Design review of the part built by this model. Coordinates are the model's own, in mm. Face numbers are marked on the shaded views. A direction names the side the tool comes from. Coordinates: 2 decimals unless noted, no trailing zeros. Loops run counter-clockwise (first coordinate to the right, second up) from the corner with the lowest first, then second, coordinate; pieces in that order, holes last. Notation, with made-up numbers: M 39,51.25 L 92,51.25 A37 cw 92,90.25 Z; hole C -4,18.25 d6. An arc over 180 degrees is marked long. Write item = value, one per line. Start each with the question number.
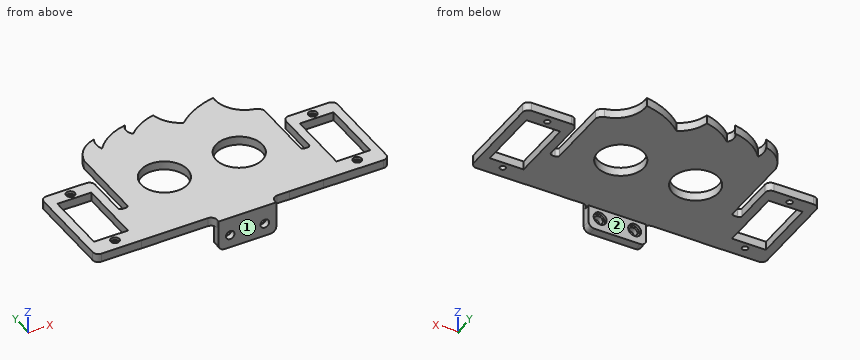
```python
from build123d import *

# Parameters (mm, degrees)
MODEL_R                 = 8.05
MODEL_R_2               = 1
MODEL_W                 = 11.8
MODEL_H                 = 22.5
SALIENTE_EXTRUIR1_DEPTH = 3
CROQUIS1_W              = 19.999999999
CROQUIS1_H              = 3
SALIENTE_EXTRUIR2_DEPTH = 8
CROQUIS2_R              = 1.5
CORTAR_EXTRUIR1_DEPTH   = 3
REDONDEO2_R             = 2
CROQUIS3_R              = 1.5
CORTAR_EXTRUIR2_DEPTH   = 1
CROQUIS4_R              = 2.25
CORTAR_EXTRUIR3_DEPTH   = 1


with BuildPart() as part:
    # Model → Saliente-Extruir1 (new body)
    with BuildSketch(Plane.XY):
        with BuildLine():
            Line((28.555278924, -36.098945331), (29.722974743, -36.098945331))
            ThreePointArc((29.722974743, -36.098945331), (30.430081524, -35.806052112), (30.722974743, -35.098945331))
            Line((30.722974743, -35.098945331), (30.722974743, -8.898603015))
            ThreePointArc((30.722974743, -8.898603015), (33.490026108, -3.637946704), (38.646410135, -0.681127156))
            ThreePointArc((38.646410135, -0.681127156), (38.00468524, -3.326803395), (38.499385848, -6.00386987))
            ThreePointArc((38.499385848, -6.00386987), (43.828182769, -1.365184752), (50.466982875, 1.051385009))
            ThreePointArc((50.466982875, 1.051385009), (49.442986911, -1.453363029), (50.490036744, -3.948561843))
            ThreePointArc((50.490036744, -3.948561843), (55.067544133, -0.573430734), (60.41559095, 1.361376528))
            ThreePointArc((60.41559095, 1.361376528), (62.493005652, -3.33729886), (66.452413363, -6.610873791))
            ThreePointArc((66.452413363, -6.610873791), (73.044296854, -2.168793623), (80.620547187, 0.236499516))
            ThreePointArc((80.620547187, 0.236499516), (82.584961535, -7.032813492), (88.968686823, -11.026544426))
            ThreePointArc((88.968686823, -11.026544426), (90.178347555, -11.787115236), (90.898959582, -13.020997464))
            Line((90.898959582, -13.020997464), (90.898959582, -35.070997464))
            ThreePointArc((90.898959582, -35.070997464), (91.191852801, -35.778104245), (91.898959582, -36.070997464))
            Line((91.898959582, -36.070997464), (92.898959582, -36.070997464))
            ThreePointArc((92.898959582, -36.070997464), (93.606066364, -35.778104245), (93.898959582, -35.070997464))
            Line((93.898959582, -35.070997464), (93.898959582, -21.120997464))
            ThreePointArc((93.898959582, -21.120997464), (94.48474602, -19.706783901), (95.898959582, -19.120997464))
            Line((95.898959582, -19.120997464), (109.698959582, -19.120997464))
            ThreePointArc((109.698959582, -19.120997464), (111.113173145, -19.706783901), (111.698959582, -21.120997464))
            Line((111.698959582, -21.120997464), (111.698959582, -51.020997464))
            ThreePointArc((111.698959582, -51.020997464), (111.113173145, -52.435211026), (109.698959582, -53.020997464))
            Line((109.698959582, -53.020997464), (88.898959583, -53.020997464))
            Line((88.898959583, -53.020997464), (76.898959583, -53.057975795))
            Line((76.898959583, -53.057975795), (72.698959583, -53.057975795))
            ThreePointArc((72.698959583, -53.057975795), (71.28474602, -53.643762233), (70.698959583, -55.057975795))
            Line((70.698959583, -55.057975795), (70.698959583, -56.057975795))
            Line((70.698959583, -56.057975795), (50.698959583, -56.057975795))
            Line((50.698959583, -56.057975795), (50.698959583, -54.961647582))
            ThreePointArc((50.698959583, -54.961647582), (50.111367037, -53.545630215), (48.6938544, -52.961654097))
            Line((48.6938544, -52.961654097), (25.611598266, -53.020573857))
            Line((25.611598266, -53.020573857), (11.698959583, -53.020573857))
            ThreePointArc((11.698959583, -53.020573857), (10.324569809, -52.451282972), (9.755278924, -51.076893199))
            Line((9.755278924, -51.076893199), (9.755278924, -21.120997464))
            ThreePointArc((9.755278924, -21.120997464), (10.341065362, -19.706783901), (11.755278924, -19.120997464))
            Line((11.755278924, -19.120997464), (25.555278924, -19.120997464))
            ThreePointArc((25.555278924, -19.120997464), (26.969492487, -19.706783901), (27.555278924, -21.120997464))
            Line((27.555278924, -21.120997464), (27.555278924, -35.098945331))
            ThreePointArc((27.555278924, -35.098945331), (27.848172143, -35.806052112), (28.555278924, -36.098945331))
        make_face()
        with Locations((73.698959582, -28.020997464)):
            Circle(MODEL_R, mode=Mode.SUBTRACT)
        with Locations((47.698959583, -28.020997464)):
            Circle(MODEL_R, mode=Mode.SUBTRACT)
        with Locations((102.798959583, -21.720997464)):
            Circle(MODEL_R_2, mode=Mode.SUBTRACT)
        with Locations((102.798959583, -49.020997464)):
            Circle(MODEL_R_2, mode=Mode.SUBTRACT)
        with Locations((18.655278924, -49.020997464)):
            Circle(MODEL_R_2, mode=Mode.SUBTRACT)
        with Locations((18.655278924, -21.720997464)):
            Circle(MODEL_R_2, mode=Mode.SUBTRACT)
        with Locations((102.798959582, -35.370997464)):
            Rectangle(MODEL_W, MODEL_H, mode=Mode.SUBTRACT)
        with Locations((18.655278924, -35.370997464)):
            Rectangle(MODEL_W, MODEL_H, mode=Mode.SUBTRACT)
    extrude(amount=SALIENTE_EXTRUIR1_DEPTH)

    # Croquis1 → Saliente-Extruir2 (add)
    with BuildSketch(Plane(origin=(0, 0, 0), x_dir=(-1, 0, 0), z_dir=(0, 0, -1))):
        with Locations((-60.698959583, -54.557975795)):
            Rectangle(CROQUIS1_W, CROQUIS1_H)
    extrude(amount=SALIENTE_EXTRUIR2_DEPTH)

    # Croquis2 → Cortar-Extruir1 (cut)
    with BuildSketch(Plane(origin=(0, -53.057975795, 0), x_dir=(1, 0, 0), z_dir=(0, 1, 0))):
        with Locations((66.698959583, 3.5)):
            Circle(CROQUIS2_R)
        with Locations((54.698959583, 3.5)):
            Circle(CROQUIS2_R)
    extrude(amount=-CORTAR_EXTRUIR1_DEPTH, mode=Mode.SUBTRACT)

    # Redondeo2
    redondeo2_edges = [part.edges().sort_by_distance(p)[0] for p in [
        (50.698959583, -54.557975795, -8),
        (70.698959583, -54.557975795, -8),
    ]]
    fillet(redondeo2_edges, radius=REDONDEO2_R)

    # Croquis3 → Cortar-Extruir2 (cut)
    with BuildSketch(Plane.XY.offset(3)):
        with Locations((18.655278924, -21.720997464)):
            Circle(CROQUIS3_R)
        with Locations((18.655278924, -49.020997464)):
            Circle(CROQUIS3_R)
        with Locations((102.798959583, -49.020997464)):
            Circle(CROQUIS3_R)
        with Locations((102.798959583, -21.720997464)):
            Circle(CROQUIS3_R)
    extrude(amount=-CORTAR_EXTRUIR2_DEPTH, mode=Mode.SUBTRACT)

    # Croquis4 → Cortar-Extruir3 (cut)
    with BuildSketch(Plane(origin=(0, -53.057975795, 0), x_dir=(1, 0, 0), z_dir=(0, 1, 0))):
        with Locations((54.698959583, 3.5)):
            Circle(CROQUIS4_R)
        with Locations((66.698959583, 3.5)):
            Circle(CROQUIS4_R)
    extrude(amount=-CORTAR_EXTRUIR3_DEPTH, mode=Mode.SUBTRACT)


solid = part.part
```
(1) Take a section at C-C (y = -45.5). State the section outline as (x, z) points.
(2) Take a section at A-A (z = -3.5). State the section outline as (x, y) points, plus the area to 3 significant figures.
(3) Take a section at B-B (x = 22). State the section outline as (y, z) points, plus the area to 3 significant figures.
(4) To check wall thickness, follow L1, parallel to X at y = -43, z = 1.75; L2, parallel to Z at x = 37, y = -14; L3, parallel to Y at x = 56.5, z = -3.25. State the ranges of each line that lie inside material, in increasing order.
(5) Take a section at D-D (x = 42.5). State the section outline as (y, z) points (3 decimals).
(6) Tool access review of the marked faces 1 and 2: name each direction out of +Z, -Z, +X, -X, +Y, -Y from which nothing blocks a thin tool from reaching the whole face with its end or side.
(7) Insertion check: pin 1 (3.5 mm diameter, centred on x = 19, y = -50, fed in from +Z); pin 2 (0.5 mm diameter, centred on x = 92.5, z = 1.5, fed in from +Y); pin 3 (5 mm diameter, centred on y = -50, z = -4.5, fed in from -X); pin 4 (0.9 mm diameter, centred on y = -20, z = 2, fed in from +X). Each pin has a flat end and moves straight along its axis. Give the tip position at first contact, or say it passes through.
Results list:
q1.outline = M 9.76,0 L 12.76,0 L 12.76,3 L 9.76,3 Z; M 24.56,0 L 96.9,0 L 96.9,3 L 24.56,3 Z; M 108.7,0 L 111.7,0 L 111.7,3 L 108.7,3 Z
q2.outline = M 50.7,-56.06 L 53.2,-56.06 L 53.2,-54.06 L 52.45,-54.06 L 52.45,-53.06 L 50.7,-53.06 Z; M 56.2,-56.06 L 65.2,-56.06 L 65.2,-54.06 L 64.45,-54.06 L 64.45,-53.06 L 56.95,-53.06 L 56.95,-54.06 L 56.2,-54.06 Z; M 68.2,-56.06 L 70.7,-56.06 L 70.7,-53.06 L 68.95,-53.06 L 68.95,-54.06 L 68.2,-54.06 Z
q2.area = 39.0 mm^2
q3.outline = M -53.02,0 L -46.62,0 L -46.62,3 L -53.02,3 Z; M -24.12,0 L -19.12,0 L -19.12,3 L -24.12,3 Z
q3.area = 34.2 mm^2
q4.L1 = 9.76 to 12.76, 24.56 to 96.9, 108.7 to 111.7
q4.L2 = 0 to 3
q4.L3 = -56.06 to -54.06
q5.outline = M -52.977,0 L -34.167,0 L -34.167,3 L -52.977,3 Z; M -21.875,0 L -2.223,0 L -2.223,3 L -21.875,3 Z
q6.face_1 = +Z, -Z, +X, -X, -Y
q6.face_2 = -Z, +X, -X, +Y
q7.pin_1 = 3
q7.pin_2 = -36.07
q7.pin_3 = through
q7.pin_4 = 111.58
